Work out the finished part from the listing and answer in its coordinate system (mm). Face numbers are marked on the shaded views. A direction names the side the tool comes from. Give positions to 0.01 mm unless a question says otherwise; leave off trailing zeros. Write each loop counter-clockwise with the first axis right and the second up, starting at its lowest first coordinate (ties: lowest second). Pieces come first, ordered by that corner, then holes. Notation, with made-up numbers: (33, 74) -> (57, 74) arc R31 cw to (57, 99) -> close; hole circle Ø11 at (69.25, 4.5). An arc over 180 degrees is marked (long way). Use a Markdown table: item, result. Add a question column.
Q1. Section D-D, the plane y = 1.5 is taken. Give the vertices of the cut face in (x, z).
Q2. Consider line 1 (Z direction, x = 35.5, y = -15.95); line 2 (X direction, y = -15.45, z = 2.5); line 3 (X direction, y = 1.3, z = -3.75). Determine where each line is inside the solid, lowest interval first.
Q3. Section C-C, the plane z = 2.5 is taken. Give the vertices of the cut face in (x, y), plus the area to 3 significant figures.
Q4. For a pull along X with two mould halves and no side action, classify the marked faces 4, 5 and 6 as pulls with the +X half, pulls with the -X half, needs draft (parallel to the pull), parting line crosses it, or undercut.
Q5. For the marked faces 1, 2 and 3, determine the directions among +Z, -Z, +X, -X, +Y, -Y from which every point of the face is accessible in a straight line to the end or side of a thin tool.
Q6. Section B-B, the plane y = -11 is taken. Give the vertices of the cut face in (x, z).
Q7. Each of these flat-tipped pins is pushed along its axis until it touches: pin 1 Ø3 at (y, z) = (-6, -3) entering from +X; pin 2 Ø1.5 at (x, z) = (-35.5, -2.5) entering from -Y; pin 3 Ø4 at (x, z) = (0, -3.75) entering from -Y; pin 4 Ø2.5 at (x, z) = (-35, -1.5) entering from +Y. Where does it stop, or does it pass through?
from build123d import *

# Parameters (mm, degrees)
SKETCH1_W           = 66
SKETCH1_H           = 5
BOSS_EXTRUDE1_DEPTH = 3
SKETCH3_W           = 3
SKETCH3_H           = 10
BOSS_EXTRUDE2_DEPTH = 14
SKETCH4_W           = 8
SKETCH4_H           = 10
BOSS_EXTRUDE3_DEPTH = 3
SKETCH5_R           = 1.22
CUT_EXTRUDE1_DEPTH  = 44.231932642
SKETCH6_R           = 1.22
CUT_EXTRUDE2_DEPTH  = 42.928510586


with BuildPart() as part:
    # Sketch1 → Boss-Extrude1 (new body)
    with BuildSketch(Plane(origin=(0, 0, 0), x_dir=(1, 0, 0), z_dir=(0, 1, 0))):
        with Locations((0, 2.5)):
            Rectangle(SKETCH1_W, SKETCH1_H)
        with Locations((0, -2.5)):
            Rectangle(SKETCH1_W, SKETCH1_H)
    extrude(amount=BOSS_EXTRUDE1_DEPTH)

    # Sketch3 → Boss-Extrude2 (add)
    with BuildSketch(Plane.XZ):
        with Locations((-31.5, 0)):
            Rectangle(SKETCH3_W, SKETCH3_H)
        with Locations((31.5, 0)):
            Rectangle(SKETCH3_W, SKETCH3_H)
    extrude(amount=BOSS_EXTRUDE2_DEPTH)

    # Sketch4 → Boss-Extrude3 (add)
    with BuildSketch(Plane.XZ.offset(14)):
        with Locations((-34, 0)):
            Rectangle(SKETCH4_W, SKETCH4_H)
        with Locations((34, 0)):
            Rectangle(SKETCH4_W, SKETCH4_H)
    extrude(amount=BOSS_EXTRUDE3_DEPTH)

    # Sketch5 → Cut-Extrude1 (cut, through all)
    with BuildSketch(Plane(origin=(0, 3, 0), x_dir=(1, 0, 0), z_dir=(0, 1, 0))):
        with Locations(Location((0, 3.75, 0), (0, 0, 270))):
            Circle(SKETCH5_R)
    extrude(amount=-CUT_EXTRUDE1_DEPTH, mode=Mode.SUBTRACT)

    # Sketch6 → Cut-Extrude2 (cut, through all)
    with BuildSketch(Plane(origin=(0, -14, 0), x_dir=(1, 0, 0), z_dir=(0, 1, 0))):
        with Locations(Location((-35.5, -2.5, 0), (0, 0, 270))):
            Circle(SKETCH6_R)
        with Locations(Location((-35.5, 2.5, 0), (0, 0, 270))):
            Circle(SKETCH6_R)
    cut_extrude2 = extrude(amount=-CUT_EXTRUDE2_DEPTH, mode=Mode.SUBTRACT)

    # Mirror1: Cut-Extrude2 across plane
    add(cut_extrude2.mirror(Plane(origin=(0, 0, 0), x_dir=(0, 0, 1), z_dir=(1, 0, 0))), mode=Mode.SUBTRACT)


solid = part.part
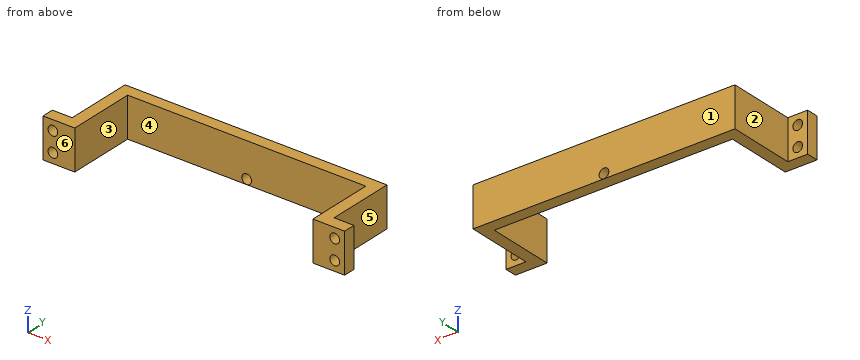
Result set:
| question | item | result |
|---|---|---|
| 1 | outline | (-33, -5) -> (33, -5) -> (33, 5) -> (-33, 5) -> close; hole circle Ø2.44 at (0, -3.75) |
| 2 | line 1 | z = -5 to -3.72, -1.28 to 1.28, 3.72 to 5 |
| 2 | line 2 | x = -38 to -36.72, -34.28 to -30, 30 to 34.28, 36.72 to 38 |
| 2 | line 3 | x = -33 to -1.22, 1.22 to 33 |
| 3 | outline | (-38, -17) -> (-36.72, -17) -> (-36.72, -14) -> (-38, -14) -> close; (-34.28, -17) -> (-30, -17) -> (-30, 0) -> (30, 0) -> (30, -17) -> (34.28, -17) -> (34.28, -14) -> (33, -14) -> (33, 3) -> (-33, 3) -> (-33, -14) -> (-34.28, -14) -> close; (36.72, -17) -> (38, -17) -> (38, -14) -> (36.72, -14) -> close |
| 3 | area | 315 mm2 |
| 4 | face 4 | undercut |
| 4 | face 5 | pulls with the +X half |
| 4 | face 6 | needs draft |
| 5 | face 1 | +Z, -Z, +X, -X, +Y |
| 5 | face 2 | +Z, -Z, -X, +Y |
| 5 | face 3 | +Z, -Z, -Y |
| 6 | outline | (-33, -5) -> (-30, -5) -> (-30, 5) -> (-33, 5) -> close; (30, -5) -> (33, -5) -> (33, 5) -> (30, 5) -> close |
| 7 | pin 1 | stops at x = 33 |
| 7 | pin 2 | passes through |
| 7 | pin 3 | stops at y = 0 |
| 7 | pin 4 | stops at y = -14 |
